Read the model definition and answer for the solid it produces. Units are mm, in the model's axes. A direction names the side the tool comes from. Round coordinates to 2 decimals unless told otherwise and drop trailing zeros. Write each loop counter-clockwise with the first axis right and the second up, starting at its lowest first coordinate (ties: lowest second). Pieces come first, ordered by that corner, then holes. Notation, with made-up numbers: (81.25, 16.25) - (140.25, 16.25) arc R33 ccw to (140.25, 50.25) - close; hole circle Ø6 at (45.5, 27). An arc over 180 degrees is marked (long way). One line per item, written item: value. Start each with the question number.
(1) A cutting plane is placed at A-A, the plane x = 6. Determine the outline of the cut face in (y, z).
(2) Find the intervals of material crossed by L1, parallel to X at y = 91, z = 39.05 (3 decimals); L2, parallel to Y at x = 6, z = 39; L3, parallel to X at y = 104, z = 41.5 (3 decimals), in increasing order.
(3) Flat-ended cylindrical pins translate along their axes: pin 1 Ø3 at (y, z) = (99, 47) entering from +X; pin 2 Ø3 at (x, z) = (24, 45) entering from -Y (3 decimals); pin 3 Ø2.5 at (x, z) = (68, 42.5) entering from +Y. Find the tip coordinate at first contact, or state that the pin passes through.
(4) For faces 1 (the face through (24, 88.985, 45)), 2 (the face through (68, 96.94, 45)), 3 (the face through (58, 124.94, 45)), determine the directions among +Z, -Z, +X, -X, +Y, -Y from which every point of the face is accessible in a straight line to the end or side of a thin tool.
(5) A cutting plane is placed at B-B, the plane z = 45.75. Determine the outline of the cut face in (x, y) (3 decimals), plus the area to 3 significant figures.
(6) A cutting plane is placed at D-D, the plane x = 56. Determine the outline of the cut face in (y, z).
(7) A cutting plane is placed at C-C, the plane y = 91. Determine the outline of the cut face in (x, z) (3 decimals).
(8) The mould has two halves that part along X. Classify faces 4 (the face through (10.13, 93, 45)), 5 (the face through (68, 124.94, 45)), 6 (the face through (4.82, 205.08, 38.79)): +X half, -X half, draft (parallel to the pull), parting line (faces both ways), or undercut.
from build123d import *

# Parameters (mm, degrees)
SKETCH009_W      = 28
SKETCH009_H      = 8.6
SKETCH009_W_2    = 8.6
SKETCH009_H_2    = 28
EXTRUDE009_DEPTH = 10
SKETCH008_W      = 77.455
SKETCH008_H      = 125
SKETCH008_R      = 1.6
EXTRUDE008_DEPTH = 1.6


with BuildPart() as extrude009:
    # Sketch009 (on Face10 of Extrude008) → Extrude009 (new body)
    with BuildSketch(Plane.XY.offset(39.6)):
        with Locations((24.13, 93.285)):
            Rectangle(SKETCH009_W, SKETCH009_H)
        with Locations((57.755, 110.94)):
            Rectangle(SKETCH009_W_2, SKETCH009_H_2)
        with Locations((68.55, 110.94)):
            Rectangle(SKETCH009_W_2, SKETCH009_H_2)
    extrude(amount=EXTRUDE009_DEPTH)


with BuildPart() as clock:
    # Sketch008 → Extrude008 (new body)
    with BuildSketch(Plane.XY.offset(38)):
        with Locations((38.7275, 147.5)):
            Rectangle(SKETCH008_W, SKETCH008_H)
        with Locations((6, 204)):
            Circle(SKETCH008_R, mode=Mode.SUBTRACT)
        with Locations((6, 91)):
            Circle(SKETCH008_R, mode=Mode.SUBTRACT)
        with Locations((71.455, 91)):
            Circle(SKETCH008_R, mode=Mode.SUBTRACT)
        with Locations((71.455, 204)):
            Circle(SKETCH008_R, mode=Mode.SUBTRACT)
    extrude(amount=EXTRUDE008_DEPTH)

    # Fusion: union Extrude009
    add(extrude009.part)


solid = clock.part
Here are the results:
1. outline: (85, 38) - (89.4, 38) - (89.4, 39.6) - (85, 39.6) - close; (92.6, 38) - (202.4, 38) - (202.4, 39.6) - (92.6, 39.6) - close; (205.6, 38) - (210, 38) - (210, 39.6) - (205.6, 39.6) - close
2. L1: 0 to 4.4, 7.6 to 69.855, 73.055 to 77.455
2. L2: 85 to 89.4, 92.6 to 202.4, 205.6 to 210
2. L3: 53.455 to 62.055, 64.25 to 72.85
3. pin 1: x = 72.85
3. pin 2: y = 88.985
3. pin 3: y = 124.94
4. face 1: +Z, +X, -X, -Y
4. face 2: +Z, +X, -Y
4. face 3: +Z, +X, -X, +Y
5. outline: (10.13, 88.985) - (38.13, 88.985) - (38.13, 97.585) - (10.13, 97.585) - close; (53.455, 96.94) - (62.055, 96.94) - (62.055, 124.94) - (53.455, 124.94) - close; (64.25, 96.94) - (72.85, 96.94) - (72.85, 124.94) - (64.25, 124.94) - close
5. area: 722 mm²
6. outline: (85, 38) - (210, 38) - (210, 39.6) - (124.94, 39.6) - (124.94, 49.6) - (96.94, 49.6) - (96.94, 39.6) - (85, 39.6) - close
7. outline: (0, 38) - (4.4, 38) - (4.4, 39.6) - (0, 39.6) - close; (7.6, 38) - (69.855, 38) - (69.855, 39.6) - (38.13, 39.6) - (38.13, 49.6) - (10.13, 49.6) - (10.13, 39.6) - (7.6, 39.6) - close; (73.055, 38) - (77.455, 38) - (77.455, 39.6) - (73.055, 39.6) - close
8. face 4: -X half
8. face 5: draft
8. face 6: undercut
